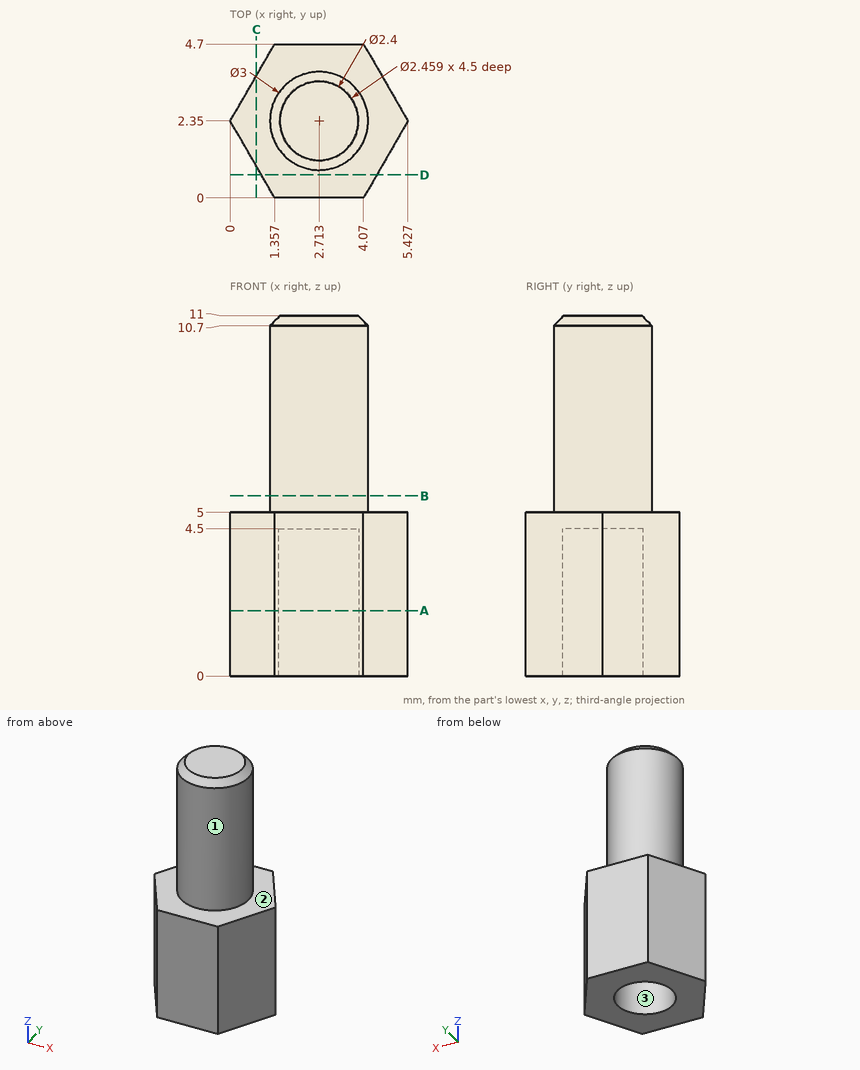
Can you work these out from the drawing? Everything is in mm from the part's minimum corner. Round coordinates to 2 decimals unless told otherwise and drop trailing zeros. Loops run counter-clockwise (first coordinate to the right, second up) from the corner with the lowest first, then second, coordinate; pieces in that order, holes last. Notation, with made-up numbers: M 38.5,36.5 L 64.5,36.5 A14 ccw 64.5,46.5 Z; hole C -26,-28 d4. An arc over 180 degrees is marked long. Write item = value, one per line.
1. Will these pins go through, and if not, where does the flat tip stop? P1, Ø1.2, axis at x = 2.5, y = 2, coming from the -Z side; P2, Ø1.5, axis at y = 1.5, z = 7.5, coming from the -X side; P3, Ø1, axis at x = 1.5, z = 7.5, coming from the +Y side.
Results below:
P1 = 4.5
P2 = 1.22
P3 = 3.67
2. Thinking about a two-plate mould opening in Y: for the marked faces 1, 2 and 3, which applies, +Y half, -Y half, draft (parallel to the pull), parting line (faces both ways), or undercut?
Results below:
face_1 = parting line
face_2 = draft
face_3 = undercut
3. I want a section at D-D, the plane y = 0.7. Write out the boundary of the cut face in (x, z) (1 decimal).
Results below:
outline = M 1,0 L 4.5,0 L 4.5,5 L 1,5 Z
4. I want a section at C-C, the plane x = 0.8. Write out the boundary of the cut face in (y, z) (1 decimal).
Results below:
outline = M 1,0 L 3.7,0 L 3.7,5 L 1,5 Z
5. I need wall thicknesses on probe 1 along Z at (x, y) = (3.4, 2.55); probe 2 along Y at (x, z) = (1.8, 2.75) (1 decimal); probe 3 along Y at (x, z) = (1.75, 2.75) (1 decimal). Which ranges of each line are inside material? Lowest first, please.
Results below:
probe_1 = 4.5 to 11
probe_2 = 0 to 1.5, 3.2 to 4.7
probe_3 = 0 to 1.6, 3.1 to 4.7
6. I want a section at B-B, the plane z = 5.5. Write out the boundary of the cut face in (x, y).
Results below:
outline = C 2.71,2.35 d3
7. I want a section at A-A, the plane z = 2. Write out the boundary of the cut face in (x, y).
Results below:
outline = M 0,2.35 L 1.36,0 L 4.07,0 L 5.43,2.35 L 4.07,4.7 L 1.36,4.7 Z; hole C 2.71,2.35 d2.46
